Source: CAD feature listing. Evaluate the final solid. Frame: model axes, mm. Give positions to 0.01 mm unless a question says otherwise; leave off trailing zeros. Loops run counter-clockwise (first coordinate to the right, second up) from the corner with the lowest first, then second, coordinate; pieces in that order, holes last. Notation, with made-up numbers: M -15,-28 L 9,-28 A25 ccw 9,-1 Z; hole C 55,76 d4. An arc over 180 degrees is marked long. Answer in a Markdown table with one row per item.
```python
from build123d import *

# Parameters (mm, degrees)
SKETCH1_R           = 1.864189773
SKETCH1_R_2         = 2
BOSS_EXTRUDE1_DEPTH = 4


with BuildPart() as part:
    # Sketch1 → Boss-Extrude1 (new body)
    with BuildSketch(Plane.XY):
        Polygon((16, 65), (16, 136), (0, 136), (0, 140), (-20, 140), (-20, 136), (-40, 136), (-40, -140), (16, -140), (16, -95), (36, -95), (36, 65), align=None)
        with Locations((2.263986992, -126.02409254)):
            Circle(SKETCH1_R, mode=Mode.SUBTRACT)
        with Locations((26, -55)):
            Circle(SKETCH1_R_2, mode=Mode.SUBTRACT)
    extrude(amount=BOSS_EXTRUDE1_DEPTH)


solid = part.part
```
1) Pin query (flat end, axial travel): pin 1 Ø3.5 at (x, y) = (2.26, -126.02) entering from -Z; pin 2 Ø1 at (x, z) = (22, 1) entering from +Y; pin 3 Ø2 at (y, z) = (95.5, 1) entering from +X; pin 4 Ø2 at (y, z) = (137.5, 1.5) entering from +X. Return the tip coordinate at first contact, or that it passes through.
Reply:
| item | result |
|---|---|
| pin 1 | passes through |
| pin 2 | stops at y = 65 |
| pin 3 | stops at x = 16 |
| pin 4 | stops at x = 0 |
2) Material intervals for L1, parallel to Y at x = 26, z = 2.1; L2, parallel to Y at x = -22.5, z = 0.6; L3, parallel to Y at x = 33, z = 1.65, sorted ascending.
Reply:
| item | result |
|---|---|
| L1 | y = -95 to -57, -53 to 65 |
| L2 | y = -140 to 136 |
| L3 | y = -95 to 65 |
3) Section A-A, the plane z = 3.2. Return loops of the section in (x, y).
Reply:
| item | result |
|---|---|
| outline | M -40,-140 L 16,-140 L 16,-95 L 36,-95 L 36,65 L 16,65 L 16,136 L 0,136 L 0,140 L -20,140 L -20,136 L -40,136 Z; hole C 2.26,-126.02 d3.73; hole C 26,-55 d4 |
